For this review, take the finished solid that the model builds, in its own axes (mm). A direction names the side the tool comes from. Give positions to 0.01 mm unless a question says otherwise; leave off trailing zeros. Order: outer loops, then holes, each group sorted by start corner. A loop starts at its lowest first (then second) coordinate and runs counter-clockwise, first axis right, second up. Notation, with made-up numbers: (60, 25.5) - (110, 25.5) arc R31 ccw to (110, 59.5) - close; hole circle Ø9 at (70, 63). An arc over 180 degrees is marked (long way). Use a Markdown table: item, result. Add a question column.
1) We need section A-A on z = -170. Write out the cut boundary in (x, y).
2) We need section B-B on y = 10. Write out the cut boundary in (x, z).
3) Clearance check with flat-ended pins moving along their axes: P1, Ø8, axis at y = 10, z = -40, coming from the -X side; P2, Ø6, axis at x = -30.5, y = 9.5, coming from the +Z side. State where each tip first meets the part, or that it passes through.
4) We need section C-C on z = -140. Write out the cut boundary in (x, y).
5) Mouldability with a two-part tool opening along Y and no side actions: class faces 1 (the face through (-5.07, 9.04, -167.69)), 2 (the face through (-20, 20, -89)), 3 (the face through (-20, 0, -89)), 4 (the face through (-5, 10, 0)) as released by +Y, released by -Y, zero draft, split by the parting line, or undercut.
6) We need section D-D on y = 3.25. Write out the cut boundary in (x, z).
7) Machinability: for faces 5 (the face through (-10, 8, -168)), 6 (the face through (-30, 10, -45)), 7 (the face through (-5, 10, -180)), 8 (the face through (-25, 10, -20)), which of the approach directions +Z, -Z, +X, -X, +Y, -Y give a long, thin tool a straight path to every point of the face, cutting with its end or side? Answer none if there is none.
8) Wall thickness on L1, parallel to Z at x = -3.5, y = 10; L2, parallel to Y at x = -25.5, z = -140; L3, parallel to Z at x = -32, y = 11.25: over which ranges is each line inside the solid? List them lowest first.
Autodesk Inventor part; units mm, degrees
ref_plane "YZ Plane" through (0, 0, 0) normal (1, 0, 0) x (0, 1, 0)
ref_plane "XZ Plane" through (0, 0, 0) normal (0, 1, 0) x (-1, 0, 0)
ref_plane "XY Plane" through (0, 0, 0) normal (0, 0, 1) x (1, 0, 0)
sketch "Эскиз1" plane through (0, 0, 0) normal (0, 1, 0) x (-1, 0, 0)
  line L0 (0, 0) -> (10, 0)
  line L1 (10, 0) -> (10, -20)
  line L2 (10, -20) -> (40, -20)
  line L3 (40, -20) -> (40, -160)
  line L4 (40, -160) -> (10, -160)
  line L5 (10, -160) -> (10, -180)
  line L6 (10, -180) -> (0, -180)
  line L7 (0, -180) -> (0, 0)
  line L8 (40, -160) -> (35, -160)
  line L9 (40, -150) -> (40, -130)
  line L10 (40, -20) -> (35, -20)
  line L11 (40, -30) -> (40, -50)
  line L12 (40, -90) -> (35, -90)
  line L13 (35, -90) -> (35, -123)
  line L14 (35, -123) -> (40, -123)
  line L15 (35, -90) -> (35, -57)
  line L16 (35, -57) -> (40, -57)
  line L17 (40, -123) -> (40, -133)
  line L18 (40, -133) -> (35, -133)
  line L19 (35, -133) -> (35, -160)
  line L20 (40, -57) -> (40, -47)
  line L21 (40, -47) -> (35, -47)
  line L22 (35, -47) -> (35, -20)
  point P0 (40, -47)
  dimension "d0" = 10
  dimension "d1" = 20
  dimension "d2" = 30
  dimension "d3" = 140
  dimension "d4" = 20
  dimension "d54" = 33
  dimension "d55" = 33
  dimension "d56" = 10
  dimension "d57" = 10
extrude "Выдавливание1" add sketch "Эскиз1" along normal blind 20
sketch "Эскиз2" plane through (-10, 0, -20) normal (-1, 0, 0) x (0, 0, 1)
  line L0 (0, 0) -> (20, 0)
  line L1 (20, 0) -> (0, 0)
  line L2 (0, 0) -> (10, 0)
  line L3 (10, 0) -> (10, 10)
  line L4 (20, 20) -> (-160, 20)
  line L5 (10, 20) -> (10, 10)
  line L6 (-140, 0) -> (-140, 20)
  line L7 (-160, 20) -> (-140, 20)
  line L8 (-140, 20) -> (-150, 20)
  line L9 (-150, 20) -> (-150, 10)
  line L10 (-150, 0) -> (-150, 10)
  circle A0 centre (10, 10) radius 2.5
  circle A1 centre (-150, 10) radius 2.5
  dimension "d7" = 10
  dimension "d10" = 10
  dimension "d12" = 5
  dimension "d14" = 5
extrude "Выдавливание2" cut sketch "Эскиз2" against normal blind 44.25
thread "Резьба4"
sketch "Эскиз3" plane through (-40, 0, -160) normal (-1, 0, 0) x (0, 0, 1)
  line L0 (140, 0) -> (140, 20)
  line L1 (140, 0) -> (140, 10)
  line L2 (140, 0) -> (70, 0)
  line L3 (160, 0) -> (-20, 0)
  line L4 (70, 10) -> (120, 10)
  line L5 (120, 10) -> (20, 10)
  line L6 (70, 10) -> (70, 0)
  circle A0 centre (120, 10) radius 5
  circle A1 centre (20, 10) radius 5
  line L7 (120, 10) -> (140, 10)
  dimension "d28" = 50
  dimension "d29" = 100
  dimension "d30" = 10
  dimension "d31" = 10
  dimension "d41" = 10
  dimension "d48" = 20
extrude "Выдавливание3" cut sketch "Эскиз3" against normal blind 20 contours A1 | L7 L4 A0 | A0 L4 L7
thread "Резьба7"
thread "Резьба8"
thread "Резьба9"
properties part number "17701729.301318.007"
Checked values:
| question | item | result |
|---|---|---|
| 1 | outline | (-10, 0) - (0, 0) - (0, 7.5) - (-10, 7.5) - close; (-10, 12.5) - (0, 12.5) - (0, 20) - (-10, 20) - close |
| 2 | outline | (-40, -160) - (-10, -160) - (-10, -167.5) - (0, -167.5) - (0, -12.5) - (-10, -12.5) - (-10, -20) - (-40, -20) - (-40, -35) - (-20, -35) - (-20, -45) - (-40, -45) - (-40, -135) - (-20, -135) - (-20, -145) - (-40, -145) - close; (-10, -180) - (0, -180) - (0, -172.5) - (-10, -172.5) - close; (-10, -7.5) - (0, -7.5) - (0, 0) - (-10, 0) - close |
| 3 | P1 | x = -20 |
| 3 | P2 | z = -20 |
| 4 | outline | (-40, 0) - (0, 0) - (0, 20) - (-40, 20) - (-40, 15) - (-20, 15) - (-20, 5) - (-40, 5) - close |
| 5 | face 1 | undercut |
| 5 | face 2 | released by +Y |
| 5 | face 3 | released by -Y |
| 5 | face 4 | zero draft |
| 6 | outline | (-40, -160) - (-10, -160) - (-10, -180) - (0, -180) - (0, 0) - (-10, 0) - (-10, -20) - (-40, -20) - close |
| 7 | face 5 | -Z, -X, +Y, -Y |
| 7 | face 6 | -X |
| 7 | face 7 | -Z, +X, -X, +Y, -Y |
| 7 | face 8 | +Z, -X, +Y, -Y |
| 8 | L1 | -180 to -172.5, -167.5 to -12.5, -7.5 to 0 |
| 8 | L2 | 0 to 5, 15 to 20 |
| 8 | L3 | -160 to -144.84, -135.16 to -44.84, -35.16 to -20 |
